Build history of the part. All positions in model axes, mm. Face numbers are marked on the shaded views. Give positions to 0.01 mm unless a question says otherwise; leave off trailing zeros. Write each loop counter-clockwise with the first axis right and the second up, starting at its lowest first coordinate (ties: lowest second). Pieces come first, ordered by that corner, then holes.
from build123d import *

# Parameters (mm, degrees)
SKETCH1_W                    = 7
SKETCH1_H                    = 10
F_8_0_8_DIAMETER_HOLE1_D     = 8
F_4_0_4_DIAMETER_HOLE1_D     = 4
F_4_0_4_DIAMETER_HOLE1_DEPTH = 17.535898385
CHAMFER1_SIZE                = 0.2


with BuildPart() as part:
    # Sketch1 → Revolve1 (revolve)
    with BuildSketch(Plane.XZ, mode=Mode.PRIVATE) as revolve1_sk:
        with Locations((3.5, 5)):
            Rectangle(SKETCH1_W, SKETCH1_H)
    revolve(revolve1_sk.sketch.rotate(Axis((0, 0, 10), (0, 0, -1)), 180), axis=Axis((0, 0, 10), (0, 0, -1)))

    # Ø8.0 (8) Diameter Hole1 (through all)
    with Locations(Plane.XY.offset(10)):
        with Locations((0, 0)):
            Hole(F_8_0_8_DIAMETER_HOLE1_D / 2)

    # Ø4.0 (4) Diameter Hole1
    with Locations(Plane(origin=(0, 7, 5), x_dir=(1, 0, 0), z_dir=(0, 1, 0))):
        with Locations((0, 0)):
            Hole(F_4_0_4_DIAMETER_HOLE1_D / 2, depth=F_4_0_4_DIAMETER_HOLE1_DEPTH)

    # Chamfer1
    chamfer1_edges = [part.edges().sort_by_distance(p)[0] for p in [
        (4, 0, 10),
        (4, 0, 0),
        (7, 0, 0),
        (7, 0, 10),
    ]]
    chamfer(chamfer1_edges, length=CHAMFER1_SIZE)


solid = part.part
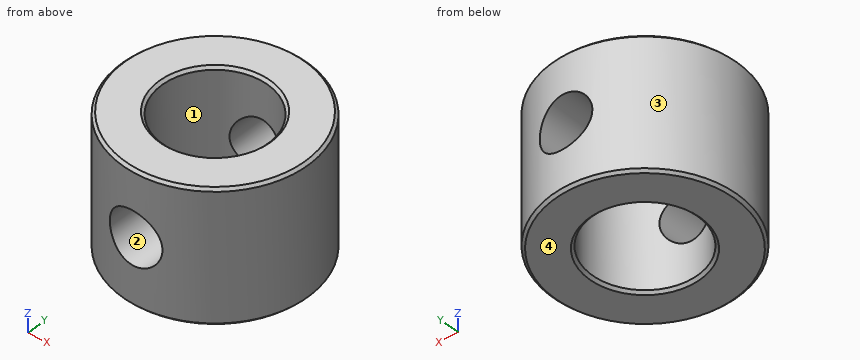
(1) Saw through at D-D, the plane z = 1.25. List the corners of the cut face in (x, y).
(2) Saw through at A-A, the plane y = 0. List the corners of the cut face in (x, z), plus the area to 3 significant figures.
(3) Saw through at C-C, the plane z = 5. List the corners of the cut face in (x, y), plus the area to 3 significant figures.
(4) Mould opens along X. For the marked faces 1, 2, 3 and 4 say: +X half, -X half, draft (parallel to the pull), parting line (faces both ways), or undercut.
(5) Probe line 1 (Z direction, x = 0, y = 5.15); line 2 (Y direction, x = 2, z = 4.25); line 3 (Y direction, x = 2.5, z = 9.25). List the from-to ranges inside material, lowest first.
(6) Saw through at B-B, the plane x = 0. List the corners of the cut face in (y, z).
(7) Drop flat-ended pins along their axis: pin 1 (7 mm diameter, centred on x = 0, y = 0, fed in from +Z); pin 2 (3 mm diameter, centred on x = 2.5, z = 1, fed in from -Y); pin 3 (3 mm diameter, centred on y = 3, z = 8.5, fed in from -X); pin 4 (2 mm diameter, centred on x = 3.5, z = 8.5, fed in from +Y). Give the stop position or say it passes through.
Computed values:
1. outline: circle Ø14 at (0, 0); hole circle Ø8 at (0, 0)
2. outline: (-7, 0.2) - (-6.8, 0) - (-4.2, 0) - (-4, 0.2) - (-4, 9.8) - (-4.2, 10) - (-6.8, 10) - (-7, 9.8) - close; (4, 0.2) - (4.2, 0) - (6.8, 0) - (7, 0.2) - (7, 9.8) - (6.8, 10) - (4.2, 10) - (4, 9.8) - close
2. area: 59.8 mm2
3. outline: (-2, -6.71) - (-2, -3.46) arc R4 cw to (-2, 3.46) - (-2, 6.71) arc R7 ccw to start; (2, -6.71) arc R7 ccw to (2, 6.71) - (2, 3.46) arc R4 cw to (2, -3.46) - close
3. area: 79.1 mm2
4. face 1: undercut
4. face 2: undercut
4. face 3: parting line
4. face 4: draft
5. line 1: z = 0 to 3, 7 to 10
5. line 2: y = -6.71 to -3.46, 3.46 to 6.71
5. line 3: y = -6.54 to -3.12, 3.12 to 6.54
6. outline: (-7, 0.2) - (-6.8, 0) - (-4.2, 0) - (-4, 0.2) - (-4, 3) - (-7, 3) - close; (-7, 7) - (-4, 7) - (-4, 9.8) - (-4.2, 10) - (-6.8, 10) - (-7, 9.8) - close; (4, 0.2) - (4.2, 0) - (6.8, 0) - (7, 0.2) - (7, 3) - (4, 3) - close; (4, 7) - (7, 7) - (7, 9.8) - (6.8, 10) - (4.2, 10) - (4, 9.8) - close
7. pin 1: passes through
7. pin 2: stops at y = -6.93
7. pin 3: stops at x = -6.84
7. pin 4: stops at y = 6.54
